from build123d import *

# Parameters (mm, degrees)
CROQUIS1_R              = 2
SALIENTE_EXTRUIR1_DEPTH = 0.75
CROQUIS2_W              = 50
CROQUIS2_H              = 20
CROQUIS2_R              = 2
SALIENTE_EXTRUIR2_DEPTH = 3.175


with BuildPart() as part:
    # Croquis1 → Saliente-Extruir1 (new, symmetric)
    with BuildSketch(Plane.XY):
        Polygon((-40, 8.85), (40, 8.85), (40, 3.1), (38.7, 3.1), (38.7, -3.1), (40, -3.1), (40, -9.85), (30, -9.85), (30, -11.15), (-30, -11.15), (-30, -8.85), (-40, -8.85), (-40, -3.75), (-37.7, -3.75), (-37.7, 3.75), (-40, 3.75), align=None)
        with Locations((20, 0)):
            Circle(CROQUIS1_R, mode=Mode.SUBTRACT)
        Circle(CROQUIS1_R, mode=Mode.SUBTRACT)
        with Locations((-20, 0)):
            Circle(CROQUIS1_R, mode=Mode.SUBTRACT)
    extrude(amount=SALIENTE_EXTRUIR1_DEPTH, both=True)

    # Croquis2 → Saliente-Extruir2 (add, symmetric)
    with BuildSketch(Plane.XY):
        with Locations((0, -1.15)):
            Rectangle(CROQUIS2_W, CROQUIS2_H)
        with Locations((-20, 0)):
            Circle(CROQUIS2_R, mode=Mode.SUBTRACT)
        Circle(CROQUIS2_R, mode=Mode.SUBTRACT)
        with Locations((20, 0)):
            Circle(CROQUIS2_R, mode=Mode.SUBTRACT)
    extrude(amount=SALIENTE_EXTRUIR2_DEPTH, both=True)


solid = part.part
The model under review builds one solid part; all positions refer to its coordinate system, in mm. A direction names the side the tool comes from. Round coordinates to 2 decimals unless told otherwise and drop trailing zeros. Loops run counter-clockwise (first coordinate to the right, second up) from the corner with the lowest first, then second, coordinate; pieces in that order, holes last. Notation, with made-up numbers: M 1,-16 L 29,-16 A16 ccw 29,13 Z; hole C 42,-2 d6. An arc over 180 degrees is marked long. Answer as a JSON object with one key per item and string values.
Item 1: We need section B-B, the plane y = 0. State the section outline as (x, z) points (3 decimals), and give its area (3 significant figures).
Check sheet entries:
{"outline": "M -37.7,-0.75 L -25,-0.75 L -25,-3.175 L -22,-3.175 L -22,3.175 L -25,3.175 L -25,0.75 L -37.7,0.75 Z; M -18,-3.175 L -2,-3.175 L -2,3.175 L -18,3.175 Z; M 2,-3.175 L 18,-3.175 L 18,3.175 L 2,3.175 Z; M 22,-3.175 L 25,-3.175 L 25,-0.75 L 38.7,-0.75 L 38.7,0.75 L 25,0.75 L 25,3.175 L 22,3.175 Z", "area": "281 mm2"}
Item 2: Clearance check with flat-ended pins moving along their axes: P1, Ø7.5, axis at x = -33, y = 3, coming from the -Z side; P2, Ø0.8, axis at y = -1, z = -0.5, coming from the -X side; P3, Ø1.6, axis at x = -36, z = 0.5, coming from the -Y side; P4, Ø12, axis at x = 30.5, y = 2, coming from the -Z side (3 decimals). State where each tip first meets the part, or that it passes through.
Check sheet entries:
{"P1": "z = -0.75", "P2": "x = -37.7", "P3": "y = -8.85", "P4": "z = -3.175"}
Item 3: The part is to be moulded in two halves that separate along Y. For faces 5 (the face through (38.7, 0, 0)), 6 (the face through (30, -10, 0)), 7 (the face through (18.4, -1.2, 0)), 8 (the face through (35, -9.85, 0)), say which applies: +Y half, -Y half, draft (parallel to the pull), parting line (faces both ways), or undercut.
Check sheet entries:
{"face 5": "undercut", "face 6": "draft", "face 7": "undercut", "face 8": "-Y half"}
Item 4: We need section C-C, the plane z = 1.5. State the section outline as (x, y) points, and give its area (3 significant figures).
Check sheet entries:
{"outline": "M -25,-11.15 L 25,-11.15 L 25,8.85 L -25,8.85 Z; hole C -20,0 d4; hole C 0,0 d4; hole C 20,0 d4", "area": "962 mm2"}
Item 5: For line 1 along Y through (x, z) = (20, -0.5); line 2 along X through (y, z) = (-1.75, 1.75); line 3 along Z through (x, y) = (-31, -5.75), list the stretches that pass through material, from the lowest coordinate up.
Check sheet entries:
{"line 1": "-11.15 to -2, 2 to 8.85", "line 2": "-25 to -20.97, -19.03 to -0.97, 0.97 to 19.03, 20.97 to 25", "line 3": "-0.75 to 0.75"}
Item 6: We need section D-D, the plane x = -34.5. State the section outline as (y, z) points, and give its area (4 significant figures).
Check sheet entries:
{"outline": "M -8.85,-0.75 L 8.85,-0.75 L 8.85,0.75 L -8.85,0.75 Z", "area": "26.55 mm2"}
Item 7: Tool access review of faces 1 (the face through (33, -1, -0.75)), 2 (the face through (39, -3.1, 0)), 3 (the face through (-25, -1, -2)), 4 (the face through (-37.7, 0, 0)): name each direction out of +Z, -Z, +X, -X, +Y, -Y from which nothing blocks a thin tool from reaching the whole face with its end or side.
Check sheet entries:
{"face 1": "-Z, +X, +Y, -Y", "face 2": "+Z, -Z, +X", "face 3": "-Z, -X, +Y, -Y", "face 4": "+Z, -Z, -X"}
Item 8: We need section A-A, the plane x = 0. State the section outline as (y, z) points (3 decimals), and give its area (3 significant figures).
Check sheet entries:
{"outline": "M -11.15,-3.175 L -2,-3.175 L -2,3.175 L -11.15,3.175 Z; M 2,-3.175 L 8.85,-3.175 L 8.85,3.175 L 2,3.175 Z", "area": "102 mm2"}
